Input: part model. Units: mm. Frame: model coordinates. Face numbers are marked on the shaded views. Coordinates: 2 decimals unless noted, no trailing zeros. Loops run counter-clockwise (first coordinate to the right, second up) from the corner with the lowest first, then second, coordinate; pieces in that order, holes last. Notation, with made-up numbers: (-29.75, 19.25) - (-21.75, 19.25) arc R7 ccw to (-21.75, 26.25) - close; hole circle Ø9 at (49, 68.5). An arc over 180 degrees is marked (long way). Use a Markdown table: item, result. Add a question column.
1. Ray query, L1, parallel to X at y = 1.2, z = 0; L2, parallel to X at y = 3, z = -1; L3, parallel to Z at x = 26.5, y = 6. Return the intervals inside material, ascending. Write a range as [from, to].
2. Section query A-A on x = 0. Return the cut outline in (y, z).
3. Section query C-C on x = -32. Return the cut outline in (y, z), then the cut area to 3 significant figures.
4. Draft query along Z for the marked faces 1, 2 and 3. Return one class per face: released by +Z, released by -Z, zero draft, split by the parting line, or undercut.
5. Contact query for flat-ended pins moving along their axis: P1, Ø3, axis at y = 9, z = 37.5, coming from the -X side; P2, Ø3.5, axis at x = 0, z = -53, coming from the +Y side; P3, Ø4, axis at y = 8.5, z = 14.5, coming from the -X side; P4, Ø1, axis at y = 5, z = 10.5, coming from the +X side. Output: stop coordinate, or through.
6. Section query B-B on z = 8.5. Return the cut outline in (x, y).
7. Section query D-D on y = 9.5. State how many separate pieces and enclosed holes the cut face has, then the cut area to 3 significant figures.
```python
from build123d import *

# Parameters (mm, degrees)
SKETCH_3_R          = 1.5
CUT_EXTRUDE_3_DEPTH = 81.099937578


with BuildPart() as part:
    # 草图2 → 旋转1 (revolve)
    with BuildSketch(Plane.XY, mode=Mode.PRIVATE) as revolve_1_sk:
        Polygon((46, 0), (46, 2), (50, 2), (50, 12), (56, 12), (56, 0), align=None)
    revolve(revolve_1_sk.sketch.rotate(Axis((0, 0, 0), (0, 1, 0)), 90), axis=Axis((0, 0, 0), (0, 1, 0)))

    # 草图3 → 切除-拉伸3 (cut, through all)
    with BuildSketch(Plane(origin=(0, 0, 0), x_dir=(1, 0, 0), z_dir=(0, 1, 0))):
        with Locations(Location((0, 53, 0), (0, 0, 270))):
            Circle(SKETCH_3_R)
        with Locations(Location((26.5, 45.899346401, 0), (0, 0, 270))):
            Circle(SKETCH_3_R)
        with Locations(Location((45.899346401, 26.5, 0), (0, 0, 270))):
            Circle(SKETCH_3_R)
        with Locations(Location((53, 0, 0), (0, 0, 270))):
            Circle(SKETCH_3_R)
        with Locations(Location((45.899346401, -26.5, 0), (0, 0, 270))):
            Circle(SKETCH_3_R)
        with Locations(Location((26.5, -45.899346401, 0), (0, 0, 270))):
            Circle(SKETCH_3_R)
        with Locations(Location((0, -53, 0), (0, 0, 270))):
            Circle(SKETCH_3_R)
        with Locations(Location((-26.5, -45.899346401, 0), (0, 0, 270))):
            Circle(SKETCH_3_R)
        with Locations(Location((-45.899346401, -26.5, 0), (0, 0, 270))):
            Circle(SKETCH_3_R)
        with Locations(Location((-53, 0, 0), (0, 0, 270))):
            Circle(SKETCH_3_R)
        with Locations(Location((-45.899346401, 26.5, 0), (0, 0, 270))):
            Circle(SKETCH_3_R)
        with Locations(Location((-26.5, 45.899346401, 0), (0, 0, 270))):
            Circle(SKETCH_3_R)
    extrude(amount=CUT_EXTRUDE_3_DEPTH, mode=Mode.SUBTRACT)


solid = part.part
```
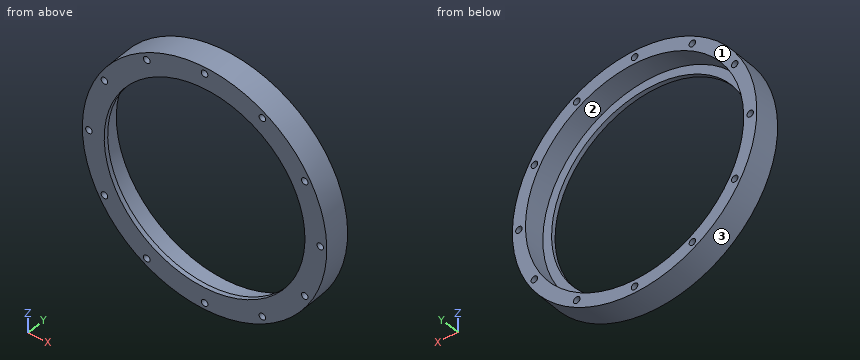
Resolved:
| question | item | result |
|---|---|---|
| 1 | L1 | [-56, -54.5], [-51.5, -46], [46, 51.5], [54.5, 56] |
| 1 | L2 | [-55.99, -54.12], [-51.88, -49.99], [49.99, 51.88], [54.12, 55.99] |
| 1 | L3 | [-49.33, -47.4], [-44.4, -42.4], [42.4, 44.4], [47.4, 49.33] |
| 2 | outline | (0, -56) - (12, -56) - (12, -54.5) - (0, -54.5) - close; (0, -51.5) - (12, -51.5) - (12, -50) - (2, -50) - (2, -46) - (0, -46) - close; (0, 46) - (2, 46) - (2, 50) - (12, 50) - (12, 51.5) - (0, 51.5) - close; (0, 54.5) - (12, 54.5) - (12, 56) - (0, 56) - close |
| 3 | outline | (0, -45.96) - (12, -45.96) - (12, -38.42) - (2, -38.42) - (2, -33.05) - (0, -33.05) - close; (0, 33.05) - (2, 33.05) - (2, 38.42) - (12, 38.42) - (12, 45.96) - (0, 45.96) - close |
| 3 | area | 202 mm² |
| 4 | face 1 | zero draft |
| 4 | face 2 | undercut |
| 4 | face 3 | split by the parting line |
| 5 | P1 | x = -42.9 |
| 5 | P2 | y = 12 |
| 5 | P3 | x = -54.59 |
| 5 | P4 | x = 55.1 |
| 6 | outline | (-55.35, 0) - (-45.21, 0) - (-45.21, 2) - (-49.27, 2) - (-49.27, 12) - (-55.35, 12) - close; (45.21, 0) - (55.35, 0) - (55.35, 12) - (49.27, 12) - (49.27, 2) - (45.21, 2) - close |
| 7 | separate pieces | 1 |
| 7 | enclosed holes | 13 |
| 7 | area | 1,910 mm² |
